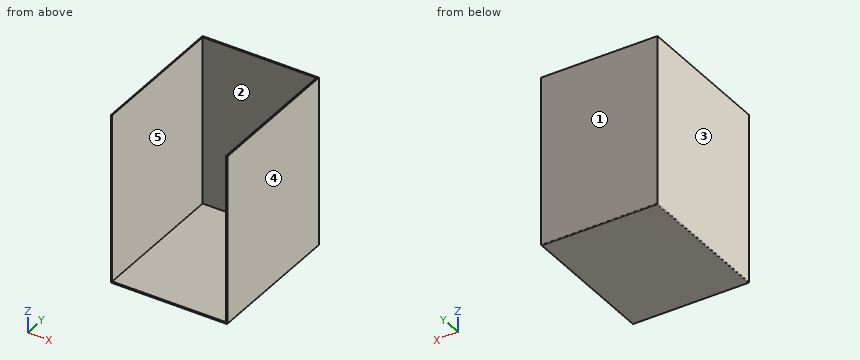
```python
from build123d import *

# Parameters (mm, degrees)
F1_DEPTH = 426
F2_W     = 295
F2_H     = 360
F3_DEPTH = 4
F4_R     = 2


# Not quite as in the source:
# - a feature names something its author has since deleted; it is built from what else it names


with BuildPart() as f1:
    # F0 (on Top) → F1 (new body)
    with BuildSketch(Plane.XY):
        Polygon((-4, -360), (0, -360), (0, 0), (-295, 0), (-295, -360), (-292.1838745495, -360), (-292.1838745495, -4), (-4, -4), align=None)
    extrude(amount=F1_DEPTH)

    # F2 (on Top) → F3 (join)
    with BuildSketch(Plane.XY):
        with Locations((-147.5, -180)):
            Rectangle(F2_W, F2_H)
    extrude(amount=-F3_DEPTH)

    # F4
    f4_edges = [f1.edges().sort_by_distance(p)[0] for p in [
        (0, -180, -4),
        (-295, -180, -4),
        (-147.5, 0, -4),
    ]]
    fillet(f4_edges, radius=F4_R)


solid = f1.part
```
Can you work these out from the model? Positions are in its coordinate system, mm. Face numbers are marked on the shaded views. A direction names the side the tool comes from. Round coordinates to 2 decimals unless told otherwise and drop trailing zeros. Loops run counter-clockwise (first coordinate to the right, second up) from the corner with the lowest first, then second, coordinate; pieces in that order, holes last. Notation, with made-up numbers: M 1,69.25 L 58,69.25 A15 cw 58,79.25 Z; hole C 54,-31.5 d9. An arc over 180 degrees is marked long. Answer as a JSON object with one key per item and string values. Group by question number.
Q1. Imagine slicing it at C-C, the plane x = -88.5. Please give me the cut outline in (y, z), then the cut area to 3 significant figures.
Q2. Please list where these lines run through material, in increasing order: L1, parallel to X at y = -265.5, z = 49; L2, parallel to Y at x = -88.5, z = 386.
Q3. We'd pull the mould along X, two halves only. Please class the marked faces 3, 4 and 5: +X half, -X half, draft (parallel to the pull), parting line (faces both ways), or undercut.
Q4. Imagine slicing it at A-A, the plane z = 296.5. Please give me the cut outline in (x, y).
Q5. Will these pins go through, and if not, where does the flat tip stop? pin 1 (1.5 mm diameter, centred on x = -71, z = 320.5, fed in from -Y); pin 2 (1.5 mm diameter, centred on x = -40, y = -66, fed in from +Z).
Q6. Imagine slicing it at B-B, the plane y = -281. Please give me the cut outline in (x, z), then the cut area to 3 significant figures.
Q7. On a 3-axis mill with a long thin cutter (end or side, diameter ignored), from which of +Z, -Z, +X, -X, +Y, -Y can I reach the whole of each face in a straight line? I mean the marked faces 1 and 2. Say none if no direction works.
Findings:
{
 "1": {"outline": "M -360,-4 L -2,-4 A2 ccw 0,-2 L 0,426 L -4,426 L -4,0 L -360,0 Z", "area": "3,140 mm2"},
 "2": {"L1": "x = -295 to -292.18, -4 to 0", "L2": "y = -4 to 0"},
 "3": {"face 3": "-X half", "face 4": "+X half", "face 5": "undercut"},
 "4": {"outline": "M -295,-360 L -292.18,-360 L -292.18,-4 L -4,-4 L -4,-360 L 0,-360 L 0,0 L -295,0 Z"},
 "5": {"pin 1": "stops at y = -4", "pin 2": "stops at z = 0"},
 "6": {"outline": "M -295,-2 A2 ccw -293,-4 L -2,-4 A2 ccw 0,-2 L 0,426 L -4,426 L -4,0 L -292.18,0 L -292.18,426 L -295,426 Z", "area": "4,080 mm2"},
 "7": {"face 1": "+Z, -Z, +X, -X, +Y", "face 2": "+Z, -Y"}
}
